For this review, use the dimensioned drawing (mm, ordinates from the lowest corner) and the shaded views. A direction names the side the tool comes from. Round coordinates to 2 decimals unless told otherwise and drop trailing zeros. Loops run counter-clockwise (first coordinate to the right, second up) from the corner with the lowest first, then second, coordinate; pieces in that order, holes last. Notation, with made-up numbers: M -38.75,21 L 18.25,21 A14 cw 18.25,38 Z; hole C 11,-28.75 d8. An arc over 180 degrees is marked long. Answer as a JSON object with one key per item and string values. Group by question number.
Item 1: Consider section C-C (x = 2.25). Give the boundary of the cut face in (y, z), and give its area (3 significant figures).
Item 2: To check wall thickness, follow line 1 (Y direction, x = 1.75, z = 1.5); line 2 (Y direction, x = 5, z = 3.5). State the ranges of each line that lie inside material, in increasing order.
Item 3: The part is to be moulded in two halves that separate along X. For the marked faces 3, 4 and 5, say which applies: +X half, -X half, draft (parallel to the pull), parting line (faces both ways), or undercut.
Item 4: Consider section D-D (z = 2.3). Give the boundary of the cut face in (x, y).
Item 5: Insertion check: P1, Ø2.5, axis at x = 7, y = 13, coming from the -Z side; P2, Ø1.7, axis at x = 6, z = 1, coming from the +Y side; P3, Ø3, axis at x = 5.207, y = 13.208, coming from the +Z side. Each pin has a flat end and moves straight along its axis. Give the tip position at first contact, or say it passes through.
Item 6: Tool access review of the marked faces 1 and 2: name each direction out of +Z, -Z, +X, -X, +Y, -Y from which nothing blocks a thin tool from reaching the whole face with its end or side.
Item 7: Consider section B-B (x = 6). Give the boundary of the cut face in (y, z).
Item 8: Consider section A-A (y = 13.5). Give the boundary of the cut face in (x, z).
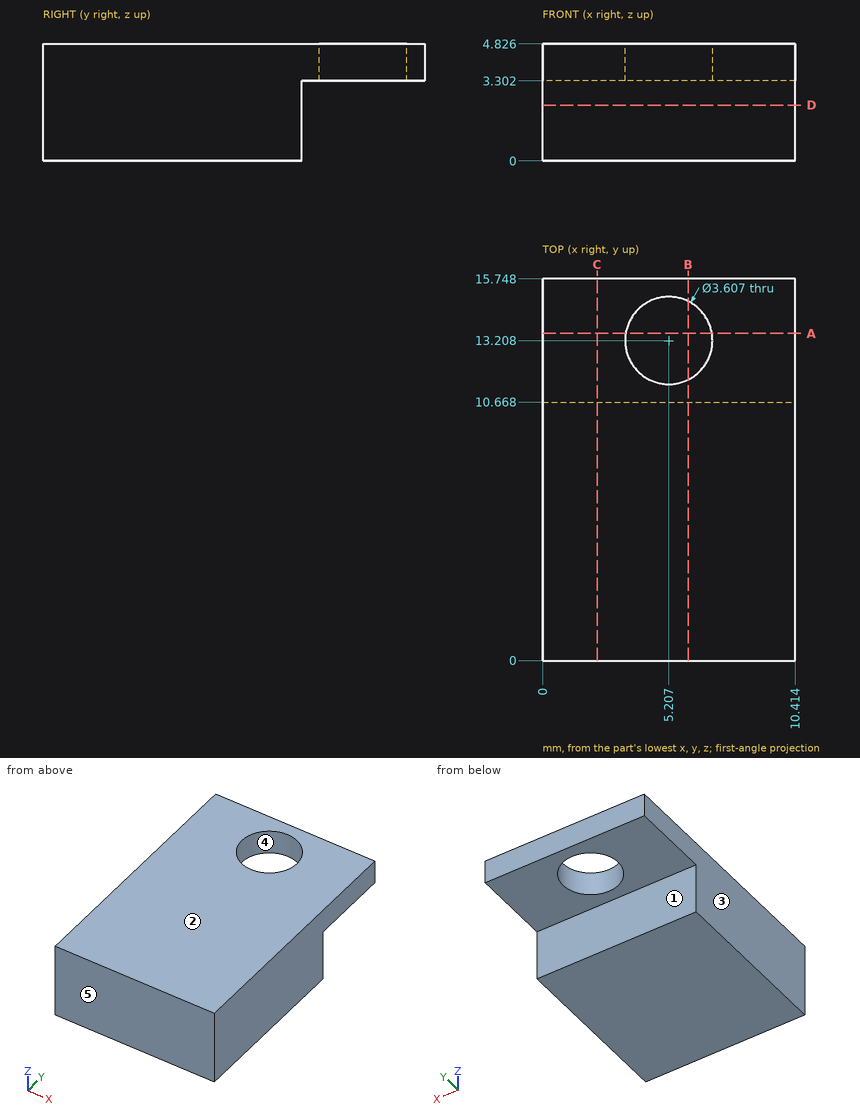
Geometry results:
{
 "1": {"outline": "M 0,0 L 10.67,0 L 10.67,3.3 L 15.75,3.3 L 15.75,4.83 L 0,4.83 Z", "area": "59.2 mm^2"},
 "2": {"line 1": "y = 0 to 10.67", "line 2": "y = 0 to 11.42, 15 to 15.75"},
 "3": {"face 3": "-X half", "face 4": "undercut", "face 5": "draft"},
 "4": {"outline": "M 0,0 L 10.41,0 L 10.41,10.67 L 0,10.67 Z"},
 "5": {"P1": "stops at z = 3.3", "P2": "stops at y = 10.67", "P3": "passes through"},
 "6": {"face 1": "-Z, +X, -X, +Y", "face 2": "+Z, +X, -X, +Y, -Y"},
 "7": {"outline": "M 0,0 L 10.67,0 L 10.67,3.3 L 11.59,3.3 L 11.59,4.83 L 0,4.83 Z; M 14.83,3.3 L 15.75,3.3 L 15.75,4.83 L 14.83,4.83 Z"},
 "8": {"outline": "M 0,3.3 L 3.43,3.3 L 3.43,4.83 L 0,4.83 Z; M 6.99,3.3 L 10.41,3.3 L 10.41,4.83 L 6.99,4.83 Z"}
}
